Geometry check sheet. Reference: the model listing, model coordinates, mm. A direction names the side the tool comes from. Give positions to 0.01 mm unless a question says otherwise; leave off trailing zeros. Order: outer loops, then holes, each group sorted by start corner. A loop starts at its lowest first (then second) coordinate and runs counter-clockwise, first axis right, second up. Notation, with made-up numbers: (-36, 45.5) - (8, 45.5) arc R24 ccw to (8, 66.5) - close; hole circle Ø9 at (-28.5, -2.75). An arc over 180 degrees is marked (long way). Put each result on its own line as item: value. Start each with the question number.
```python
from build123d import *

# Parameters (mm, degrees)
F0_W     = 25
F0_H     = 25
F1_DEPTH = 10
F4_W     = 25
F4_H     = 25
F4_R     = 4.5
F5_DEPTH = 20
F6_R     = 6
F7_DEPTH = 40


with BuildPart() as f1:
    # F0 (on Top) → F1 (new body)
    with BuildSketch(Plane.XY):
        Rectangle(F0_W, F0_H)
    extrude(amount=F1_DEPTH)

    # F2 (on Front) → F3 (revolve, cut)
    with BuildSketch(Plane.XZ):
        Polygon((4.5, 0), (0, 8), (0, 0), align=None)
    revolve(axis=Axis((0, 0, 4), (0, 0, -1)), mode=Mode.SUBTRACT)

    # F4 (on Top) → F5 (join)
    with BuildSketch(Plane.XY):
        Rectangle(F4_W, F4_H)
        Circle(F4_R, mode=Mode.SUBTRACT)
    extrude(amount=-F5_DEPTH)

    # F6 (on face) → F7 (join)
    with BuildSketch(Plane.XY.offset(10)):
        Circle(F6_R)
    extrude(amount=F7_DEPTH)


solid = f1.part
```
Item 1: Cross-section at B-B (x = -7.5). Enter the section's corners in (y, z), and give its area (3 significant figures).
Item 2: Set-up check for faces 1 (the face through (-6, 0, 30)), 2 (the face through (0, 6, -20)), 3 (the face through (-0.59, 4.46, -9.86)): record each of +Z, -Z, +X, -X, +Y, -Y from which the full face is reachable in a straight line by a thin tool's end or side.
Item 3: Release check for a two-part mould opening along Y. For faces 4 (the face through (0, 12.5, -5)), 5 (the face through (0, 0, 50)), 6 (the face through (-0.37, 1.68, 4.94)) record: +Y half, -Y half, draft (parallel to the pull), parting line (faces both ways), or undercut.
Item 4: Cross-section at A-A (z = -3). Enter the section's corners in (x, y), and give its area (3 significant figures).
Item 5: Gauge pin test, flat ends, axial feed: pin 1 Ø8 at (x, y) = (0, 0) entering from -Z; pin 2 Ø3 at (x, y) = (8, -5.5) entering from +Z; pin 3 Ø2 at (x, z) = (3.5, 23) entering from +Y. Record the tip position at first contact, or that the pin passes through.
Item 6: Thickness scan on line 1 along X through (y, z) = (-0.25, -11); line 2 along Y through (x, z) = (0, -15.5); line 3 along Z through (x, y) = (3.5, -5.75). Record the ranges inside material, lowest first.
Recorded:
1. outline: (-12.5, -20) - (12.5, -20) - (12.5, 10) - (-12.5, 10) - close
1. area: 750 mm^2
2. face 1: +Z
2. face 2: -Z, +X, -X, +Y, -Y
2. face 3: -Z
3. face 4: +Y half
3. face 5: draft
3. face 6: undercut
4. outline: (-12.5, -12.5) - (12.5, -12.5) - (12.5, 12.5) - (-12.5, 12.5) - close; hole circle Ø9 at (0, 0)
4. area: 561 mm^2
5. pin 1: stops at z = 0.89
5. pin 2: stops at z = 10
5. pin 3: stops at y = 5.45
6. line 1: x = -12.5 to -4.49, 4.49 to 12.5
6. line 2: y = -12.5 to -4.5, 4.5 to 12.5
6. line 3: z = -20 to 10
